Work out the finished part from the listing and answer in its coordinate system (mm). A direction names the side the tool comes from. Coordinates: 2 decimals unless noted, no trailing zeros. Loops run counter-clockwise (first coordinate to the right, second up) from the corner with the lowest first, then second, coordinate; pieces in that order, holes last. Notation, with made-up numbers: (36.5, 41.5) -> (44.5, 41.5) arc R30 ccw to (44.5, 80.5) -> close; hole circle Ø3 at (-26, -15). An arc over 180 degrees is marked (long way). One line per question, with ' | ' between items.
```python
from build123d import *

# Parameters (mm, degrees)
PAD_DEPTH           = 12
SKETCH001_W         = 1.6
SKETCH001_H         = 12
PAD001_DEPTH        = 4.1
LINEARPATTERN_COUNT = 2
LINEARPATTERN_PITCH = 28.1
PAD002_DEPTH        = 3.6
SKETCH004_R         = 1.95
PAD003_DEPTH        = 3.5
SKETCH005_R         = 1
PAD004_DEPTH        = 1.2
FILLET_R            = 2
FILLET001_R         = 2
FILLET002_R         = 2
FILLET003_R         = 2
SKETCH006_R         = 1
POCKET_DEPTH        = 16.901


with BuildPart() as part:
    # Sketch → Pad (new body)
    with BuildSketch(Plane.XY):
        Polygon((-19, 20.4), (5, 20.4), (5, 3), (0, 0), (-19, 0), align=None)
    extrude(amount=PAD_DEPTH)

    # Sketch001 → Pad001 (new body)
    with BuildSketch(Plane.YZ.offset(5)):
        with Locations((16.1, 6)):
            Rectangle(SKETCH001_W, SKETCH001_H)
    pad001 = extrude(amount=PAD001_DEPTH)

    # LinearPattern: Pad001 ×2
    with Locations(*[(-i * LINEARPATTERN_PITCH, 0, 0) for i in range(1, LINEARPATTERN_COUNT)]):
        add(pad001)

    # Sketch003 → Pad002 (new body)
    with BuildSketch(Plane(origin=(0, 20.4, 0), x_dir=(-1, 0, 0), z_dir=(0, 1, 0))):
        with BuildLine():
            ThreePointArc((6.017699, 9.289787), (-5, 6), (6.017699, 2.710213))
            ThreePointArc((6.017699, 2.710213), (10, 6), (6.017699, 9.289787))
        make_face()
    extrude(amount=PAD002_DEPTH)

    # Sketch004 → Pad003 (new body)
    with BuildSketch(Plane(origin=(0, 24, 0), x_dir=(-1, 0, 0), z_dir=(0, 1, 0))):
        with Locations((1, 6)):
            Circle(SKETCH004_R)
    extrude(amount=PAD003_DEPTH)

    # Sketch005 → Pad004 (new body)
    with BuildSketch(Plane(origin=(0, 24, 0), x_dir=(-1, 0, 0), z_dir=(0, 1, 0))):
        with Locations((6.65, 6)):
            Circle(SKETCH005_R)
    extrude(amount=PAD004_DEPTH)

    # Fillet
    fillet_edges = [part.edges().sort_by_distance(p)[0] for p in [
        (9.1, 16.1, 12),
    ]]
    fillet(fillet_edges, radius=FILLET_R)

    # Fillet001
    fillet001_edges = [part.edges().sort_by_distance(p)[0] for p in [
        (-23.1, 16.1, 12),
    ]]
    fillet(fillet001_edges, radius=FILLET001_R)

    # Fillet002
    fillet002_edges = [part.edges().sort_by_distance(p)[0] for p in [
        (9.1, 16.1, 0),
    ]]
    fillet(fillet002_edges, radius=FILLET002_R)

    # Fillet003
    fillet003_edges = [part.edges().sort_by_distance(p)[0] for p in [
        (-23.1, 16.1, 0),
    ]]
    fillet(fillet003_edges, radius=FILLET003_R)

    # Sketch006 → Pocket (cut, through all)
    with BuildSketch(Plane(origin=(0, 16.9, 0), x_dir=(-1, 0, 0), z_dir=(0, 1, 0))):
        with Locations((-7, 6)):
            Circle(SKETCH006_R)
        with Locations((21, 6)):
            Circle(SKETCH006_R)
    extrude(amount=-POCKET_DEPTH, mode=Mode.SUBTRACT)


solid = part.part
```
1) The mould has two halves that part along Z. Classify faces 1 (the face through (5, 22, 6)), 2 (the face through (-22.5, 16.11, 11.43)), 3 (the face through (-21, 16, 7)): released by +Z, released by -Z, zero draft, split by the parting line, or undercut.
Check values:
face 1: split by the parting line | face 2: released by +Z | face 3: undercut
2) Find section C-C (y = 6.5). Write down the section's boundary in (x, z).
Check values:
outline: (-19, 0) -> (5, 0) -> (5, 12) -> (-19, 12) -> close
3) Find the intervals of material crossed by line 1 along Z through (x, y) = (-21, 16.55); line 2 along Y through (x, z) = (-4, 9.5); line 3 along Y through (x, z) = (8, 3), in increasing order.
Check values:
line 1: z = 0 to 5, 7 to 12 | line 2: y = 0 to 24 | line 3: y = 15.3 to 16.9
4) For faces 4 (the face through (-19.7, 15.3, 5.9)), 5 (the face through (5, 19, 6)), 6 (the face through (5, 9, 6)), 7 (the face through (-19.7, 16.9, 5.9)), determine the directions among +Z, -Z, +X, -X, +Y, -Y from which every point of the face is accessible in a straight line to the end or side of a thin tool.
Check values:
face 4: +Z, -Z, -X, -Y | face 5: +Z, -Z, +X, +Y | face 6: +Z, -Z, +X, -Y | face 7: +Z, -Z, -X, +Y
5) Flat-ended cylindrical pins translate along their axes: pin 1 (3.5 mm diameter, centred on x = -8, z = 4, fed in from +Y); pin 2 (1.7 mm diameter, centred on y = 19, z = 7.5, fed in from -X); pin 3 (5 mm diameter, centred on y = 3, z = 4.5, fed in from +X). Find the tip coordinate at first contact, or state that the pin passes through.
Check values:
pin 1: stops at y = 25.2 | pin 2: stops at x = -19 | pin 3: stops at x = 5
6) Find section A-A (x = -6.65). Write down the section's boundary in (y, z), plus the area to 3 significant figures.
Check values:
outline: (0, 0) -> (20.4, 0) -> (20.4, 2.65) -> (24, 2.65) -> (24, 5) -> (25.2, 5) -> (25.2, 7) -> (24, 7) -> (24, 9.35) -> (20.4, 9.35) -> (20.4, 12) -> (0, 12) -> close | area: 271 mm^2
7) Find section D-D (x = 3.5). Write down the section's boundary in (y, z), plus the area to 3 significant figures.
Check values:
outline: (2.1, 0) -> (20.4, 0) -> (20.4, 2.03) -> (24, 2.03) -> (24, 9.97) -> (20.4, 9.97) -> (20.4, 12) -> (2.1, 12) -> close | area: 248 mm^2
8) Find section B-B (z = 10.5). Write down the section's boundary in (x, y).
Check values:
outline: (-23.04, 15.3) -> (-19, 15.3) -> (-19, 0) -> (0, 0) -> (5, 3) -> (5, 15.3) -> (9.04, 15.3) -> (9.04, 16.9) -> (5, 16.9) -> (5, 20.4) -> (2.97, 20.4) -> (2.97, 24) -> (-4.97, 24) -> (-4.97, 20.4) -> (-19, 20.4) -> (-19, 16.9) -> (-23.04, 16.9) -> close
